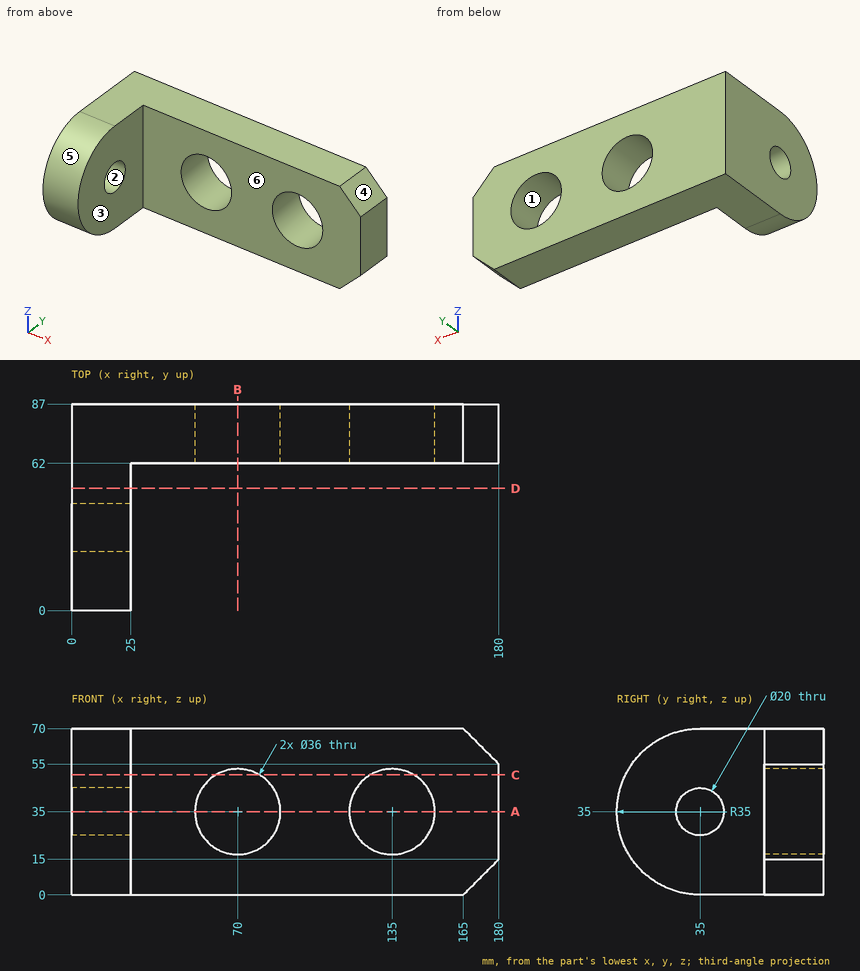
Part print with two shaded views. Sizes in mm from the minimum x, y, z corner. A direction names the side the tool comes from. Round coordinates to 2 decimals unless told otherwise and drop trailing zeros. Loops run counter-clockwise (first coordinate to the right, second up) from the corner with the lowest first, then second, coordinate; pieces in that order, holes last.
Item 1: Pin check, flat tips, straight feed: P1, Ø2, axis at y = 46, z = 40.5, coming from the +X side; P2, Ø6, axis at x = 58.5, z = 60, coming from the -Y side. Stop position of each tip, or through.
Item 2: Saw through at D-D (y = 51.5). List the corners of the cut face in (x, z).
Item 3: Which spindle directions (+Z, -Z, +X, -X, +Y, -Y) get a long thin tool onto all of the face, cutting with end or side? Do the marked faces 5 and 6. Say none if no direction does.
Item 4: Saw through at C-C (z = 50.5). List the corners of the cut face in (x, y).
Item 5: Saw through at B-B (x = 70). List the corners of the cut face in (y, z).
Item 6: Two-plate mould, pull along Z, no slides. Class the marked faces 1, 2, 3 and 4: released by +Z, released by -Z, zero draft, split by the parting line, or undercut.
Item 7: Drill centre lines: line 1 along Z through (x, y) = (135, 75); line 2 along Z through (x, y) = (9, 35); line 3 along Y through (x, z) = (104, 51.5). Where is each one in solid material? Low to high.
Item 8: Saw through at A-A (z = 35). List the corners of the cut face in (x, y), then the cut area to 3 significant figures.
Worked answers:
1. P1: stops at x = 25
1. P2: stops at y = 62
2. outline: (0, 0) - (25, 0) - (25, 70) - (0, 70) - close
3. face 5: +X, -X, -Y
3. face 6: +Z, -Z, +X, -Y
4. outline: (0, 3.62) - (25, 3.62) - (25, 62) - (60.85, 62) - (60.85, 87) - (0, 87) - close; (79.15, 62) - (125.85, 62) - (125.85, 87) - (79.15, 87) - close; (144.15, 62) - (180, 62) - (180, 87) - (144.15, 87) - close
5. outline: (62, 0) - (87, 0) - (87, 17) - (62, 17) - close; (62, 53) - (87, 53) - (87, 70) - (62, 70) - close
6. face 1: undercut
6. face 2: undercut
6. face 3: zero draft
6. face 4: released by +Z
7. line 1: z = 0 to 17, 53 to 70
7. line 2: z = 0 to 25, 45 to 70
7. line 3: y = 62 to 87
8. outline: (0, 0) - (25, 0) - (25, 25) - (0, 25) - close; (0, 45) - (25, 45) - (25, 62) - (52, 62) - (52, 87) - (0, 87) - close; (88, 62) - (117, 62) - (117, 87) - (88, 87) - close; (153, 62) - (180, 62) - (180, 87) - (153, 87) - close
8. area: 3,750 mm2
